```python
from build123d import *

# Parameters (mm, degrees)
SKETCH1_W           = 133.35
SKETCH1_H           = 254
SKETCH1_R           = 1.5
SKETCH1_W_2         = 113.35
SKETCH1_H_2         = 234
BOSS_EXTRUDE1_DEPTH = 3.175


with BuildPart() as part:
    # Sketch1 → Boss-Extrude1 (new body)
    with BuildSketch(Plane.XY):
        with Locations((66.675, 127)):
            Rectangle(SKETCH1_W, SKETCH1_H)
        with Locations((5, 5)):
            Circle(SKETCH1_R, mode=Mode.SUBTRACT)
        with Locations((5, 249)):
            Circle(SKETCH1_R, mode=Mode.SUBTRACT)
        with Locations((5, 127)):
            Circle(SKETCH1_R, mode=Mode.SUBTRACT)
        with Locations((128.35, 249)):
            Circle(SKETCH1_R, mode=Mode.SUBTRACT)
        with Locations((128.35, 127)):
            Circle(SKETCH1_R, mode=Mode.SUBTRACT)
        with Locations((128.35, 5)):
            Circle(SKETCH1_R, mode=Mode.SUBTRACT)
        with Locations((66.675, 127)):
            Rectangle(SKETCH1_W_2, SKETCH1_H_2, mode=Mode.SUBTRACT)
    extrude(amount=BOSS_EXTRUDE1_DEPTH)


solid = part.part
```
Check sheet for the modelled part. Datum: model origin and axes. Units: mm. Coordinates: 2 decimals unless noted, no trailing zeros. Loops run counter-clockwise (first coordinate to the right, second up) from the corner with the lowest first, then second, coordinate; pieces in that order, holes last.
1) Sectioned sample at A-A (x = 85). Record the boundary of the cut face in (y, z) (3 decimals).
2) Gauge pin test, flat end, axial feed: pin 1 (2.5 mm diameter, centred on x = 128.35, y = 5, fed in from -Z). Record the tip position at first contact, or that the pin passes through.
3) Material ranges on probe 1 along Y at (x, z) = (128.35, 1.7); probe 2 along X at (y, z) = (249, 1.6); probe 3 along X at (y, z) = (127, 2.45), recorded low to high.
4) Sectioned sample at C-C (y = 75). Record the boundary of the cut face in (x, z) (3 decimals).
5) Sectioned sample at B-B (z = 1.6). Record the boundary of the cut face in (x, y).
Check sheet entries:
1. outline: (0, 0) - (10, 0) - (10, 3.175) - (0, 3.175) - close; (244, 0) - (254, 0) - (254, 3.175) - (244, 3.175) - close
2. pin 1: passes through
3. probe 1: y = 0 to 3.5, 6.5 to 125.5, 128.5 to 247.5, 250.5 to 254
3. probe 2: x = 0 to 3.5, 6.5 to 126.85, 129.85 to 133.35
3. probe 3: x = 0 to 3.5, 6.5 to 10, 123.35 to 126.85, 129.85 to 133.35
4. outline: (0, 0) - (10, 0) - (10, 3.175) - (0, 3.175) - close; (123.35, 0) - (133.35, 0) - (133.35, 3.175) - (123.35, 3.175) - close
5. outline: (0, 0) - (133.35, 0) - (133.35, 254) - (0, 254) - close; hole circle Ø3 at (5, 5); hole circle Ø3 at (5, 127); hole circle Ø3 at (5, 249); hole (10, 10) - (123.35, 10) - (123.35, 244) - (10, 244) - close; hole circle Ø3 at (128.35, 5); hole circle Ø3 at (128.35, 127); hole circle Ø3 at (128.35, 249)
